Could you check a few things on this model? Use its own coordinates, in mm. Coordinates: 2 decimals unless noted, no trailing zeros. Write each loop counter-clockwise with the first axis right and the second up, starting at its lowest first coordinate (ties: lowest second). Pieces come first, ordered by that corner, then holes.
```python
from build123d import *

# Parameters (mm, degrees)
SKETCH1_W           = 100
SKETCH1_H           = 100
BOSS_EXTRUDE1_DEPTH = 5


with BuildPart() as part:
    # Sketch1 → Boss-Extrude1 (new body)
    with BuildSketch(Plane(origin=(0, 0, 0), x_dir=(1, 0, 0), z_dir=(0, 1, 0))):
        Rectangle(SKETCH1_W, SKETCH1_H)
    extrude(amount=BOSS_EXTRUDE1_DEPTH)

    # Sketch4 → Ø5.0mm Dowel Hole1 (revolve, cut)
    with BuildSketch(Plane(origin=(40, 5, 40), x_dir=(0, 0, 1), z_dir=(1, 0, 0))):
        Polygon((0, 0), (0, 5), (2.525, 5), (2.5, 4.975), (2.5, 0), align=None)
    f_5_0mm_dowel_hole1 = revolve(axis=Axis((40, 11.35, 40), (0, -1, 0)), mode=Mode.SUBTRACT)

    # Mirror1: Ø5.0mm Dowel Hole1 across plane
    add(f_5_0mm_dowel_hole1.mirror(Plane(origin=(0, 0, 0), x_dir=(0, 0, 1), z_dir=(1, 0, 0))), mode=Mode.SUBTRACT)

    # Mirror1 at the second plane: Ø5.0mm Dowel Hole1 across plane
    add(f_5_0mm_dowel_hole1.mirror(Plane.XY), mode=Mode.SUBTRACT)

    # Mirror1 at the second plane copy 1 sketc → Mirror1 at the second plane copy 1 (revolve, cut)
    with BuildSketch(Plane(origin=(-40, 5, -40), x_dir=(0, 0, -1), z_dir=(-1, 0, 0))):
        Polygon((0, 0), (0, 5), (2.525, 5), (2.5, 4.975), (2.5, 0), align=None)
    revolve(axis=Axis((-40, 11.35, -40), (0, -1, 0)), mode=Mode.SUBTRACT)


solid = part.part
```
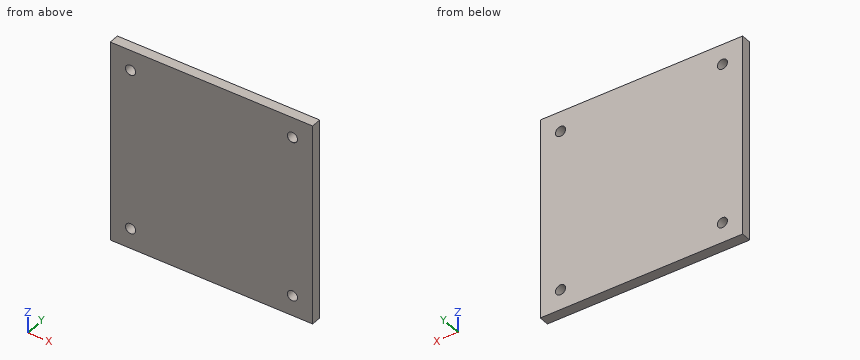
1. I want a section at B-B on z = 40. Please give me the cut outline in (x, y) (3 decimals), plus the area to 3 significant figures.
Verdict:
outline: (-50, 0) - (-42.525, 0) - (-42.5, 0.025) - (-42.5, 5) - (-50, 5) - close; (-37.5, 0.025) - (-37.475, 0) - (37.475, 0) - (37.5, 0.025) - (37.5, 5) - (-37.5, 5) - close; (42.5, 0.025) - (42.525, 0) - (50, 0) - (50, 5) - (42.5, 5) - close
area: 450 mm2
2. I want a section at A-A on x = 40. Please give me the cut outline in (y, z) (3 decimals).
Verdict:
outline: (0, -50) - (5, -50) - (5, -42.5) - (0.025, -42.5) - (0, -42.525) - close; (0, -37.475) - (0.025, -37.5) - (5, -37.5) - (5, 37.5) - (0.025, 37.5) - (0, 37.475) - close; (0, 42.525) - (0.025, 42.5) - (5, 42.5) - (5, 50) - (0, 50) - close
3. Please list where these lines run through material, in increasing order: line 1 along X through (y, z) = (2.05, -40); line 2 along X through (y, z) = (2.4, 39.5).
Verdict:
line 1: x = -50 to -42.5, -37.5 to 37.5, 42.5 to 50
line 2: x = -50 to -42.45, -37.55 to 37.55, 42.45 to 50
